Build history of the part. All positions in model axes, mm. A direction names the side the tool comes from. Give positions to 0.01 mm unless a question says otherwise; leave off trailing zeros. Order: outer loops, then holes, each group sorted by start corner. A loop starts at its lowest first (then second) coordinate and runs counter-clockwise, first axis right, second up. Notation, with made-up numbers: (55.25, 16) - (107.25, 16) arc R11 cw to (107.25, 32) - close; hole circle Ø7 at (23, -32.5). An arc over 180 degrees is marked (long way). Write each question's results on one line, items separated by ' | '. Start each with the question number.
from build123d import *

# Parameters (mm, degrees)
BOSS_EXTRU_1_DEPTH      = 3
ESQUISSE3_W             = 105
ESQUISSE3_H             = 60
ESQUISSE3_W_2           = 101
ESQUISSE3_H_2           = 56
BOSS_EXTRU_2_DEPTH      = 30
CONG_2_R                = 2
CONG_4_R                = 2
ESQUISSE4_W             = 26
ESQUISSE4_H             = 14
ENL_V_MAT_EXTRU_2_DEPTH = 162
ESQUISSE6_W             = 18
ESQUISSE6_H             = 30
BOSS_EXTRU_7_DEPTH      = 6.5


with BuildPart() as part:
    # Esquisse2 → Boss.-Extru.1 (new body)
    with BuildSketch(Plane(origin=(0, 0, 0), x_dir=(1, 0, 0), z_dir=(0, 1, 0))):
        Polygon((0, 30), (-52.5, 30), (-52.5, -30), (0, -30), (52.5, -30), (52.5, 30), align=None)
    extrude(amount=BOSS_EXTRU_1_DEPTH)

    # Esquisse3 → Boss.-Extru.2 (add)
    with BuildSketch(Plane(origin=(0, 3, 0), x_dir=(1, 0, 0), z_dir=(0, 1, 0))):
        Rectangle(ESQUISSE3_W, ESQUISSE3_H)
        Rectangle(ESQUISSE3_W_2, ESQUISSE3_H_2, mode=Mode.SUBTRACT)
    extrude(amount=BOSS_EXTRU_2_DEPTH)

    # Congé2
    cong_2_edges = [part.edges().sort_by_distance(p)[0] for p in [
        (52.5, 16.5, -30),
        (52.5, 16.5, 30),
        (-52.5, 16.5, 30),
        (-52.5, 16.5, -30),
    ]]
    fillet(cong_2_edges, radius=CONG_2_R)

    # Congé4
    cong_4_edges = [part.edges().sort_by_distance(p)[0] for p in [
        (-50.5, 18, 28),
        (50.5, 18, 28),
        (50.5, 18, -28),
        (-50.5, 18, -28),
    ]]
    fillet(cong_4_edges, radius=CONG_4_R)

    # Esquisse4 → Enlèv. mat.-Extru.2 (cut)
    with BuildSketch(Plane.ZY.offset(52.5)):
        with Locations((-1, 16.5)):
            Rectangle(ESQUISSE4_W, ESQUISSE4_H)
    extrude(amount=-ENL_V_MAT_EXTRU_2_DEPTH, mode=Mode.SUBTRACT)

    # Esquisse6 → Boss.-Extru.7 (add)
    with BuildSketch(Plane(origin=(0, 3, 0), x_dir=(1, 0, 0), z_dir=(0, 1, 0))):
        with Locations((-41.5, 1)):
            Rectangle(ESQUISSE6_W, ESQUISSE6_H)
    boss_extru_7 = extrude(amount=BOSS_EXTRU_7_DEPTH)

    # Symétrie1: Boss.-Extru.7 across plane
    add(boss_extru_7.mirror(Plane(origin=(0, 0, 0), x_dir=(0, 0, 1), z_dir=(1, 0, 0))))


solid = part.part
Item 1: Cut at C-C, the plane x = -13. List the corners of the cut face in (y, z).
Item 2: Cut at B-B, the plane y = 13. List the corners of the cut face in (x, z).
Item 3: Cut at A-A, the plane z = 9. List the corners of the cut face in (x, y).
Item 4: Two-plate mould, pull along Y, no slides. Class faces 1 (the flat face through (51, 16, 12)), 2 (the flat face through (32.5, 6, -1)), 3 (the flat face through (-1, 0, 0)): +Y half, -Y half, draft (parallel to the pull), parting line (faces both ways), or undercut.
Item 5: Which spindle directions (+Z, -Z, +X, -X, +Y, -Y) get a long thin tool onto all of the face, cutting with end or side? Do faces 4 (the flat face through (-32.5, 6, -1)), 5 (the flat face through (-52.5, 24, 0)). Say none if no direction does.
Item 6: Flat gauge pins, fed straight in: pin 1 Ø10 at (x, z) = (38.5, -5.5) entering from +Y; pin 2 Ø0.6 at (x, y) = (51, 18) entering from -Z; pin 3 Ø1.6 at (x, y) = (51.5, 15.5) entering from +Z. Where does each tip first touch, or does it go through?
Item 7: Probe line 1 along Z through (x, y) = (13, 13); line 2 along X through (y, z) = (28, 12); line 3 along Y through (x, z) = (-11, 0.5). List the from-to ranges inside material, lowest first. Write a range as from..to.
Item 8: Cut at D-D, the plane z = 22. List the corners of the cut face in (x, y).
Values found:
1) outline: (0, -30) - (33, -30) - (33, -28) - (3, -28) - (3, 28) - (33, 28) - (33, 30) - (0, 30) - close
2) outline: (-52.5, -28) arc R2 ccw to (-50.5, -30) - (50.5, -30) arc R2 ccw to (52.5, -28) - (52.5, -14) - (50.5, -14) - (50.5, -26) arc R2 cw to (48.5, -28) - (-48.5, -28) arc R2 cw to (-50.5, -26) - (-50.5, -14) - (-52.5, -14) - close; (-52.5, 12) - (-50.5, 12) - (-50.5, 26) arc R2 cw to (-48.5, 28) - (48.5, 28) arc R2 cw to (50.5, 26) - (50.5, 12) - (52.5, 12) - (52.5, 28) arc R2 ccw to (50.5, 30) - (-50.5, 30) arc R2 ccw to (-52.5, 28) - close
3) outline: (-52.5, 0) - (52.5, 0) - (52.5, 9.5) - (32.5, 9.5) - (32.5, 3) - (-32.5, 3) - (-32.5, 9.5) - (-52.5, 9.5) - close; (-52.5, 23.5) - (-50.5, 23.5) - (-50.5, 33) - (-52.5, 33) - close; (50.5, 23.5) - (52.5, 23.5) - (52.5, 33) - (50.5, 33) - close
4) face 1: undercut | face 2: draft | face 3: -Y half
5) face 4: +Y | face 5: +Z, -Z, -X, +Y, -Y
6) pin 1: stops at y = 9.5 | pin 2: stops at z = -29.99 | pin 3: stops at z = 29.99
7) line 1: z = -30..-28, 28..30 | line 2: x = -52.5..-50.5, 50.5..52.5 | line 3: y = 0..3
8) outline: (-52.5, 0) - (52.5, 0) - (52.5, 33) - (50.5, 33) - (50.5, 3) - (-50.5, 3) - (-50.5, 33) - (-52.5, 33) - close
